For this review, use the dimensioned drawing (mm, ordinates from the lowest corner) and the shaded views. A direction names the side the tool comes from. Round coordinates to 2 decimals unless told otherwise and drop trailing zeros. Write each loop counter-clockwise with the first axis right and the second up, starting at its lowest first coordinate (ties: lowest second). Pieces come first, ordered by that corner, then holes.
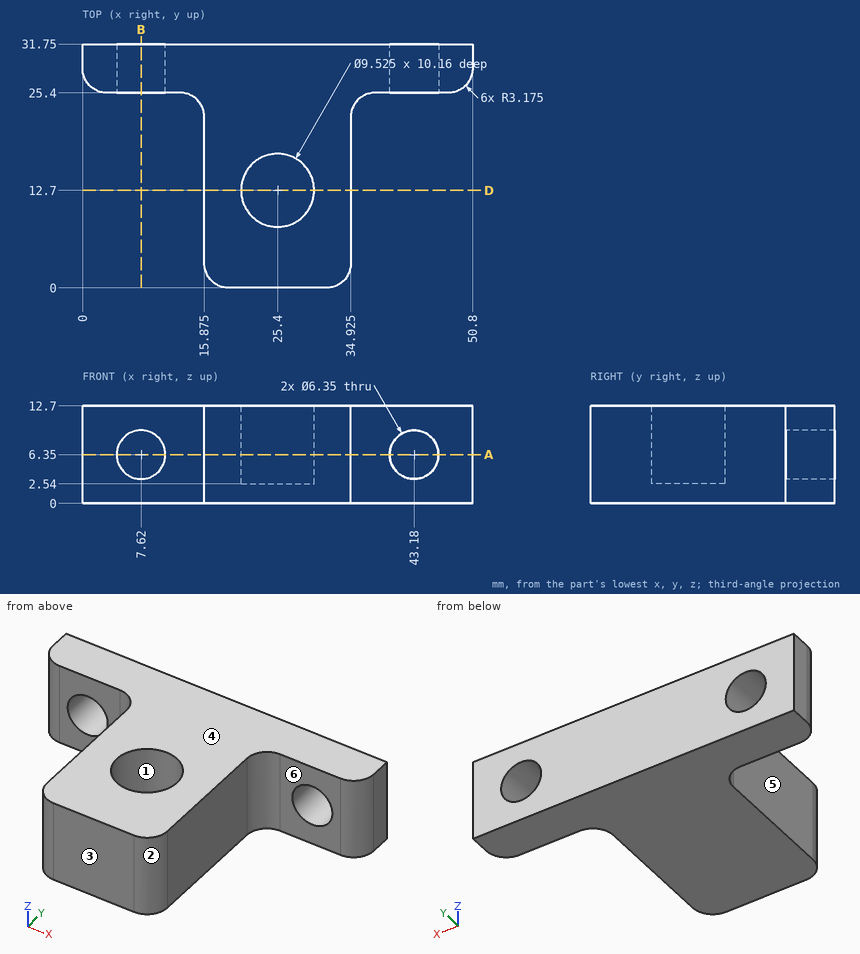
1) Add section B-B on x = 7.62. State the section outline as (y, z) points (3 decimals).
2) The part is to be moulded in two halves that separate along X. For the marked faces 1, 2 and 3, say which applies: pulls with the +X half, pulls with the -X half, needs draft (parallel to the pull), parting line crosses it, or undercut.
3) For the marked faces 4, 5 and 6, list the 3-axis set-ups (+Z, -Z, +X, -X, +Y, -Y) from which the entire face can be reached by the end or side of a thin tool; tool diameter is ignored.
4) Add section D-D on y = 12.7. State the section outline as (x, z) points (1 decimal).
5) For P1, Ø3, axis at x = 44.5, z = 8.5, coming from the -Y side; P2, Ø6, axis at y = 11.5, z = 5.5, coming from the +X side (3 decimals); P3, Ø2, axis at y = 22.5, z = 8.5, coming from the +X side, all flat-tipped, find the tip position at first contact; note any pin that passes through.
6) For line 1 along X through (y, z) = (27.5, 8.25); line 2 along X through (y, z) = (12.7, 5.75) (1 decimal); line 3 along X through (y, z) = (5, 1) (3 decimals), list the stretches that pass through material, from the lowest coordinate up.
7) Add section A-A on z = 6.35. Count the separate pieces of the cut face and the enclosed holes in it, and give its area (3 significant figures).
Computed:
1. outline: (25.4, 0) - (31.75, 0) - (31.75, 3.175) - (25.4, 3.175) - close; (25.4, 9.525) - (31.75, 9.525) - (31.75, 12.7) - (25.4, 12.7) - close
2. face 1: undercut
2. face 2: pulls with the +X half
2. face 3: needs draft
3. face 4: +Z, +X, -X, +Y, -Y
3. face 5: +Z, -Z, -X, -Y
3. face 6: +Z, -Z, +X, -Y
4. outline: (15.9, 0) - (34.9, 0) - (34.9, 12.7) - (30.2, 12.7) - (30.2, 2.5) - (20.6, 2.5) - (20.6, 12.7) - (15.9, 12.7) - close
5. P1: stops at y = 25.4
5. P2: stops at x = 34.925
5. P3: stops at x = 35.19
6. line 1: x = 0.19 to 5.08, 10.16 to 40.64, 45.72 to 50.61
6. line 2: x = 15.9 to 20.6, 30.2 to 34.9
6. line 3: x = 15.875 to 34.925
7. separate pieces: 3
7. enclosed holes: 1
7. area: 650 mm2
